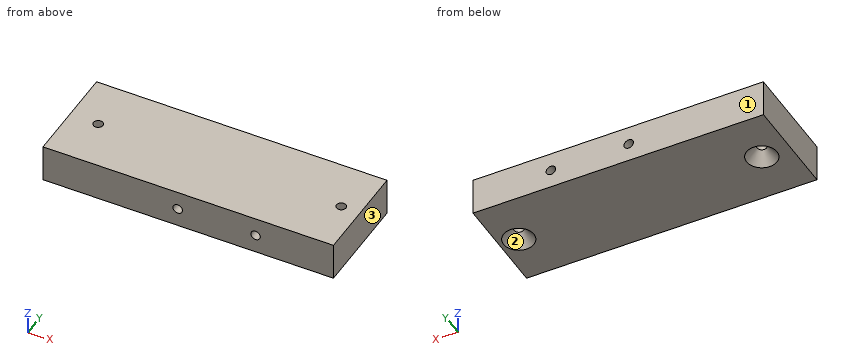
from build123d import *

# Parameters (mm, degrees)
SKETCH1_W           = 97.3
SKETCH1_H           = 33.95
BOSS_EXTRUDE1_DEPTH = 12.7
HOLE1_D             = 3.175
HOLE1_DEPTH         = 31.75
HOLE1_CSINK_D       = 10.16
HOLE1_CSINK_ANGLE   = 82
HOLE1_TIP           = 0.953866233
HOLE2_D             = 3.175
HOLE2_DEPTH         = 31.75
HOLE2_CSINK_D       = 10.16
HOLE2_CSINK_ANGLE   = 82
HOLE2_TIP           = 0.953866233
HOLE5_D             = 3.175
HOLE5_DEPTH         = 31.75
HOLE5_CSINK_D       = 10.16
HOLE5_CSINK_ANGLE   = 82
HOLE5_TIP           = 0.953866233
HOLE6_D             = 3.175
HOLE6_DEPTH         = 31.75
HOLE6_CSINK_D       = 10.16
HOLE6_CSINK_ANGLE   = 82
HOLE6_TIP           = 0.953866233


with BuildPart() as part:
    # Sketch1 → Boss-Extrude1 (new body)
    with BuildSketch(Plane.XY):
        with Locations((-292.654465963, -36.025)):
            Rectangle(SKETCH1_W, SKETCH1_H)
    extrude(amount=-BOSS_EXTRUDE1_DEPTH)

    # Hole1
    with Locations(Plane(origin=(-124.004465969, 0, -10.424290059), x_dir=(-1, 0, 0), z_dir=(0, 1, 0))):
        with Locations((126.349999994, 161.374290059), (146.083333327, 4.074290059), (172.166666661, 4.074290059), (126.349999994, 34.524290059), (126.349999994, 130.924290059), (-172.166666661, 4.074290059), (-146.083333327, 4.074290059), (-126.349999994, 34.524290059), (-126.349999994, 130.924290059), (-126.349999994, 161.374290059)):
            CounterSinkHole(HOLE1_D / 2, HOLE1_CSINK_D / 2, depth=HOLE1_DEPTH, counter_sink_angle=HOLE1_CSINK_ANGLE)
            with Locations((0, 0, -(HOLE1_DEPTH + HOLE1_TIP / 2))):  # 118° drill point
                Cone(0, HOLE1_D / 2, HOLE1_TIP, mode=Mode.SUBTRACT)

    # Hole2
    with Locations(Plane(origin=(-124.004465969, -72.05, -10.424290059), x_dir=(1, 0, 0), z_dir=(0, -1, 0))):
        with Locations((126.349999994, 161.374290059), (146.083333327, 4.074290059), (172.166666661, 4.074290059), (126.349999994, 34.524290059), (126.349999994, 130.924290059), (-172.166666661, 4.074290059), (-146.083333327, 4.074290059), (-126.349999994, 34.524290059), (-126.349999994, 130.924290059), (-126.349999994, 161.374290059)):
            CounterSinkHole(HOLE2_D / 2, HOLE2_CSINK_D / 2, depth=HOLE2_DEPTH, counter_sink_angle=HOLE2_CSINK_ANGLE)
            with Locations((0, 0, -(HOLE2_DEPTH + HOLE2_TIP / 2))):  # 118° drill point
                Cone(0, HOLE2_D / 2, HOLE2_TIP, mode=Mode.SUBTRACT)

    # Hole5
    with Locations(Plane(origin=(-124.004465969, -208.286738577, -12.7), x_dir=(-1, 0, 0), z_dir=(0, 0, -1))):
        with Locations((207.774999994, 172.261738577), (126.349999994, 172.261738577)):
            CounterSinkHole(HOLE5_D / 2, HOLE5_CSINK_D / 2, depth=HOLE5_DEPTH, counter_sink_angle=HOLE5_CSINK_ANGLE)
            with Locations((0, 0, -(HOLE5_DEPTH + HOLE5_TIP / 2))):  # 118° drill point
                Cone(0, HOLE5_D / 2, HOLE5_TIP, mode=Mode.SUBTRACT)

    # Hole6
    with Locations(Plane(origin=(-124.004465969, -6.35, -10.424290059), x_dir=(-1, 0, 0), z_dir=(0, 1, 0))):
        with Locations((-207.774999994, 333.02141023), (-207.774999994, 225.48903684), (-207.774999994, 137.424290059), (-172.166666661, 4.074290059), (-146.083333327, 4.074290059), (-94.599999994, 161.374290059), (94.599999994, 161.374290059), (146.083333327, 4.074290059), (172.166666661, 4.074290059), (207.774999994, 137.424290059), (207.774999994, 225.48903684), (207.774999994, 333.02141023), (166.795833328, 301.970350905), (40.979166666, 301.970350905), (-40.979166666, 301.970350905), (-166.795833328, 301.970350905), (0, 193.124290059), (0, 301.970350905), (0, 412.366411751), (-126.349999994, 106.824290059), (-126.349999994, 58.624290059), (126.349999994, 58.624290059), (126.349999994, 106.824290059)):
            CounterSinkHole(HOLE6_D / 2, HOLE6_CSINK_D / 2, depth=HOLE6_DEPTH, counter_sink_angle=HOLE6_CSINK_ANGLE)
            with Locations((0, 0, -(HOLE6_DEPTH + HOLE6_TIP / 2))):  # 118° drill point
                Cone(0, HOLE6_D / 2, HOLE6_TIP, mode=Mode.SUBTRACT)


solid = part.part
Work out the finished part from the listing and answer in its coordinate system (mm). Face numbers are marked on the shaded views. Round coordinates to 2 decimals unless told otherwise and drop trailing zeros. Use one line per item in the form item = value.
(1) Flat-ended cylindrical pins translate along their axes: P1, Ø1.9, axis at x = -296.17, z = -6.35, coming from the +Y side; P2, Ø3, axis at x = -270.09, z = -6.35, coming from the -Y side; P3, Ø3, axis at x = -270.09, z = -6.35, coming from the +Y side. Find the tip coordinate at first contact, or state that the pin passes through.
Answer list:
P1 = -38.48
P2 = -40.25
P3 = -38.15
(2) Straight lines are drawn through the part: line 1 (X direction, y = -47.25, z = -6.35); line 2 (Z direction, x = -296, y = -48.5); line 3 (X direction, y = -24, z = -6.75). For each, find the intervals that lie inside material, in ascending order.
Answer list:
line_1 = -341.3 to -297.76, -294.58 to -271.68, -268.5 to -244
line_2 = -12.7 to -7.93, -4.77 to 0
line_3 = -341.3 to -297.71, -294.63 to -271.62, -268.55 to -244
(3) For a pull along Y with two mould halves and no side action, classify the marked faces 1, 2 and 3 as released by +Y, released by -Y, zero draft, split by the parting line, or undercut.
Answer list:
face_1 = released by +Y
face_2 = undercut
face_3 = zero draft
